Input: part model. Units: mm. Frame: model coordinates. Face numbers are marked on the shaded views. A direction names the side the tool comes from. Coordinates: 2 decimals unless noted, no trailing zeros. Loops run counter-clockwise (first coordinate to the right, second up) from the corner with the lowest first, then second, coordinate; pieces in that order, holes last. Notation, with made-up numbers: (0.5, 83) - (55.5, 83) arc R19 cw to (55.5, 105) - close; hole circle Ø3 at (-34.5, -12.5). An arc over 180 degrees is marked (long way). Use a Markdown table: item, result. Add a question column.
1. Contact query for flat-ended pins moving along their axis: P1, Ø6, axis at x = -51, z = 42, coming from the +Y side; P2, Ø0.8, axis at x = -39.5, y = 7, coming from the -Z side; P3, Ø4, axis at x = 30, y = 14, coming from the +Z side; P4, Ø1.7, axis at x = -45.5, z = 34.5, coming from the +Y side. Output: stop coordinate, or through.
2. Draft query along X for the marked faces 4, 5 and 6. Return one class per face: released by +X, released by -X, zero draft, split by the parting line, or undercut.
3. Section query C-C on y = 1.75. Return the cut outline in (x, z), then the cut area to 3 significant figures.
4. Ray query, L1, parallel to Y at x = -30, z = 0.8; L2, parallel to X at y = 5.5, z = 28.5; L3, parallel to Y at x = -49.5, z = 32.5. Return the intervals inside material, ascending. Write a range as [from, to].
5. Section query B-B on y = 14. State how many separate pieces and enclosed holes the cut face has, then the cut area to 3 significant figures.
6. Section query A-A on z = 16. Return the cut outline in (x, y).
7. Access query for the marked faces 1, 2 and 3. Directions: +Z, -Z, +X, -X, +Y, -Y. A direction counts if a zero-diameter tool reaches every point of the face in a straight line with its end or side. Return the directions, or none.
```python
from build123d import *

# Parameters (mm, degrees)
SKETCH_1_W          = 110
SKETCH_1_H          = 20
SKETCH_1_R          = 1.7
EXTRUDE_1_DEPTH     = 4.5
SKETCH_2_W          = 20
SKETCH_2_H          = 8
EXTRUDE_2_DEPTH     = 45
CUT_EXTRUDE_1_DEPTH = 1.3
CUT_EXTRUDE_2_DEPTH = 29
SKETCH_11_R         = 1.7
CUT_EXTRUDE_3_DEPTH = 167
CUT_EXTRUDE_4_DEPTH = 1.5


with BuildPart() as part:
    # 草图1 → 凸台-拉伸1 (new body)
    with BuildSketch(Plane.XY):
        with Locations((0, 10)):
            Rectangle(SKETCH_1_W, SKETCH_1_H)
        with Locations((-45, 14)):
            Circle(SKETCH_1_R, mode=Mode.SUBTRACT)
        with Locations((-30, 14)):
            Circle(SKETCH_1_R, mode=Mode.SUBTRACT)
        with Locations((-15, 14)):
            Circle(SKETCH_1_R, mode=Mode.SUBTRACT)
        with Locations((15, 14)):
            Circle(SKETCH_1_R, mode=Mode.SUBTRACT)
        with Locations((30, 14)):
            Circle(SKETCH_1_R, mode=Mode.SUBTRACT)
        with Locations((45, 14)):
            Circle(SKETCH_1_R, mode=Mode.SUBTRACT)
    extrude(amount=EXTRUDE_1_DEPTH)

    # 草图2 → 凸台-拉伸2 (add)
    with BuildSketch(Plane.XY.offset(4.5)):
        with Locations((-45, 4)):
            Rectangle(SKETCH_2_W, SKETCH_2_H)
        with Locations((45, 4)):
            Rectangle(SKETCH_2_W, SKETCH_2_H)
    extrude(amount=EXTRUDE_2_DEPTH)

    # 草图3 → 切除-拉伸1 (cut)
    with BuildSketch(Plane.XY.offset(4.5)):
        Polygon((-45, 17.22), (-47.7886018, 15.61), (-47.7886018, 12.39), (-45, 10.78), (-42.2113982, 12.39), (-42.2113982, 15.61), align=None)
        Polygon((-30, 17.22), (-32.7886018, 15.61), (-32.7886018, 12.39), (-30, 10.78), (-27.2113982, 12.39), (-27.2113982, 15.61), align=None)
        Polygon((-15, 17.22), (-17.7886018, 15.61), (-17.7886018, 12.39), (-15, 10.78), (-12.2113982, 12.39), (-12.2113982, 15.61), align=None)
        Polygon((15, 17.22), (12.2113982, 15.61), (12.2113982, 12.39), (15, 10.78), (17.7886018, 12.39), (17.7886018, 15.61), align=None)
        Polygon((30, 17.22), (27.2113982, 15.61), (27.2113982, 12.39), (30, 10.78), (32.7886018, 12.39), (32.7886018, 15.61), align=None)
        Polygon((45, 17.22), (42.2113982, 15.61), (42.2113982, 12.39), (45, 10.78), (47.7886018, 12.39), (47.7886018, 15.61), align=None)
    extrude(amount=-CUT_EXTRUDE_1_DEPTH, mode=Mode.SUBTRACT)

    # 草图10 → 切除-拉伸2 (cut)
    with BuildSketch(Plane.XZ):
        Polygon((0, 0), (10.1, 0), (10.1, 2.1), (-10.1, 2.1), (-10.1, 0), align=None)
    extrude(amount=-CUT_EXTRUDE_2_DEPTH, mode=Mode.SUBTRACT)

    # 草图11 → 切除-拉伸3 (cut)
    with BuildSketch(Plane.XZ):
        with Locations((-331.768706014, -207.641629986)):
            Circle(SKETCH_11_R)
        with Locations((-337.768706014, -197.641629986)):
            Circle(SKETCH_11_R)
        with Locations((-325.768706014, -197.641629986)):
            Circle(SKETCH_11_R)
        with Locations((-247.768706014, -197.641629986)):
            Circle(SKETCH_11_R)
        with Locations((-235.768706014, -197.641629986)):
            Circle(SKETCH_11_R)
        with Locations((-241.768706014, -207.641629986)):
            Circle(SKETCH_11_R)
    extrude(amount=-CUT_EXTRUDE_3_DEPTH, mode=Mode.SUBTRACT)

    # 草图12 → 切除-拉伸4 (cut)
    with BuildSketch(Plane(origin=(0, 8, 0), x_dir=(1, 0, 0), z_dir=(0, 1, 0))):
        Polygon((-41.78, -33.5), (-43.39, -30.7113982), (-46.61, -30.7113982), (-48.22, -33.5), (-46.61, -36.2886018), (-43.39, -36.2886018), align=None)
        Polygon((-47.78, -43.5), (-49.39, -40.7113982), (-52.61, -40.7113982), (-54.22, -43.5), (-52.61, -46.2886018), (-49.39, -46.2886018), align=None)
        Polygon((-35.78, -43.5), (-37.39, -40.7113982), (-40.61, -40.7113982), (-42.22, -43.5), (-40.61, -46.2886018), (-37.39, -46.2886018), align=None)
        Polygon((37.39, -46.2886018), (35.78, -43.5), (37.39, -40.7113982), (40.61, -40.7113982), (42.22, -43.5), (40.61, -46.2886018), align=None)
        Polygon((49.39, -46.2886018), (47.78, -43.5), (49.39, -40.7113982), (52.61, -40.7113982), (54.22, -43.5), (52.61, -46.2886018), align=None)
        Polygon((43.39, -36.2886018), (41.78, -33.5), (43.39, -30.7113982), (46.61, -30.7113982), (48.22, -33.5), (46.61, -36.2886018), align=None)
    extrude(amount=-CUT_EXTRUDE_4_DEPTH, mode=Mode.SUBTRACT)


solid = part.part
```
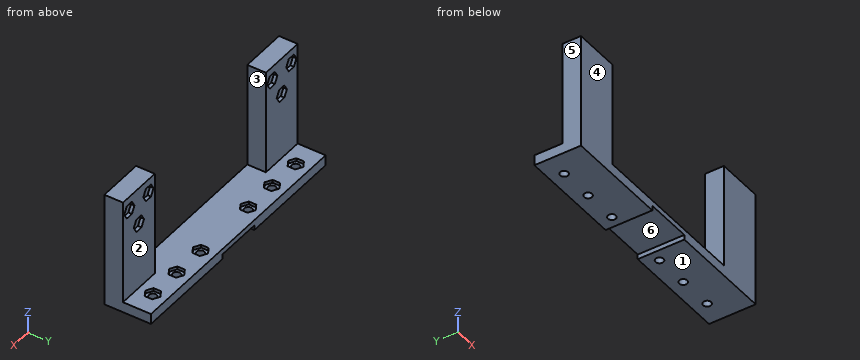
Resolved:
| question | item | result |
|---|---|---|
| 1 | P1 | y = 8 |
| 1 | P2 | z = 0 |
| 1 | P3 | z = 3.2 |
| 1 | P4 | y = 6.5 |
| 2 | face 4 | zero draft |
| 2 | face 5 | released by -X |
| 2 | face 6 | undercut |
| 3 | outline | (-55, 0) - (-10.1, 0) - (-10.1, 2.1) - (10.1, 2.1) - (10.1, 0) - (55, 0) - (55, 49.5) - (35, 49.5) - (35, 4.5) - (-35, 4.5) - (-35, 49.5) - (-55, 49.5) - close |
| 3 | area | 2,250 mm² |
| 4 | L1 | [0, 12.3], [15.7, 20] |
| 4 | L2 | [-55, -35], [35, 55] |
| 4 | L3 | [0, 8] |
| 5 | separate pieces | 7 |
| 5 | enclosed holes | 0 |
| 5 | area | 344 mm² |
| 6 | outline | (-55, 0) - (-35, 0) - (-35, 8) - (-55, 8) - close; (35, 0) - (55, 0) - (55, 8) - (35, 8) - close |
| 7 | face 1 | -Z, +X, -X, +Y, -Y |
| 7 | face 2 | +Z, +X, -X, +Y |
| 7 | face 3 | +Z, +Y, -Y |
